from build123d import *

# Parameters (mm, degrees)
SKETCH1_W           = 7.62
SKETCH1_H           = 7.62
BOSS_EXTRUDE1_DEPTH = 10.16
SKETCH2_W           = 7.62
SKETCH2_H           = 7.62
SKETCH2_R           = 1.905
CUT_EXTRUDE1_DEPTH  = 7.62
FILLET1_R           = 2.54
FILLET2_R           = 2.54
FILLET3_R           = 2.54
FILLET4_R           = 2.54


with BuildPart() as part:
    # Sketch1 → Boss-Extrude1 (new body)
    with BuildSketch(Plane(origin=(0, 0, 0), x_dir=(1, 0, 0), z_dir=(0, 1, 0))):
        with Locations((3.81, 3.81)):
            Rectangle(SKETCH1_W, SKETCH1_H)
    extrude(amount=BOSS_EXTRUDE1_DEPTH)

    # Sketch2 → Cut-Extrude1 (cut)
    with BuildSketch(Plane(origin=(0, 10.16, 0), x_dir=(1, 0, 0), z_dir=(0, 1, 0))):
        with Locations((3.81, 3.81)):
            Rectangle(SKETCH2_W, SKETCH2_H)
        with Locations(Location((3.81, 3.81, 0), (0, 0, 270))):
            Circle(SKETCH2_R, mode=Mode.SUBTRACT)
    extrude(amount=-CUT_EXTRUDE1_DEPTH, mode=Mode.SUBTRACT)

    # Fillet1
    fillet1_edges = [part.edges().sort_by_distance(p)[0] for p in [
        (7.62, 1.27, -7.62),
    ]]
    fillet(fillet1_edges, radius=FILLET1_R)

    # Fillet2
    fillet2_edges = [part.edges().sort_by_distance(p)[0] for p in [
        (0, 1.27, -7.62),
    ]]
    fillet(fillet2_edges, radius=FILLET2_R)

    # Fillet3
    fillet3_edges = [part.edges().sort_by_distance(p)[0] for p in [
        (7.62, 1.27, 0),
    ]]
    fillet(fillet3_edges, radius=FILLET3_R)

    # Fillet4
    fillet4_edges = [part.edges().sort_by_distance(p)[0] for p in [
        (0, 1.27, 0),
    ]]
    fillet(fillet4_edges, radius=FILLET4_R)


solid = part.part
Geometry check sheet. Reference: the model listing, model coordinates, mm. A direction names the side the tool comes from. Coordinates: 2 decimals unless noted, no trailing zeros. Order: outer loops, then holes, each group sorted by start corner. A loop starts at its lowest first (then second) coordinate and runs counter-clockwise, first axis right, second up. Notation, with made-up numbers: (-2, -19.75) -> (16, -19.75) arc R28 ccw to (16, 11.25) -> close; hole circle Ø5 at (18.25, 83). An arc over 180 degrees is marked (long way). Use a Markdown table: item, result. Add a question column.
1. Cross-section at D-D (z = -6.75). Enter the section's corners in (x, y), and give its area (3 significant figures).
2. Go/stop test with flat-tipped pins: pin 1 Ø2 at (x, y) = (3, 3.5) entering from +Z; pin 2 Ø1.5 at (x, y) = (1, 8) entering from +Z; pin 3 Ø3 at (y, z) = (3.5, -6.5) entering from -X. Record where each tip stops, or that it passes through.
3. Cross-section at B-B (x = 3.81). Enter the section's corners in (y, z) (3 decimals), and give its area (3 significant figures).
4. Set-up check for faces 1 (the face through (4, 1, 0)), 2 (the face through (5, 2.54, -6)): record each of +Z, -Z, +X, -X, +Y, -Y from which the full face is reachable in a straight line by a thin tool's end or side.
5. Cross-section at A-A (y = 1.25). Enter the section's corners in (x, z).
6. Cross-section at C-C (y = 4.75). Enter the section's corners in (x, z) (3 decimals).
7. Material ranges on L1, parallel to Y at x = 0.5, z = -2.5; L2, parallel to X at y = 1.75, z = -6.5; L3, parallel to X at y = 8, z = -4.75, recorded low to high.
Filled sheet:
| question | item | result |
|---|---|---|
| 1 | outline | (0.63, 0) -> (6.99, 0) -> (6.99, 2.54) -> (0.63, 2.54) -> close |
| 1 | area | 16.2 mm2 |
| 2 | pin 1 | z = 0 |
| 2 | pin 2 | through |
| 2 | pin 3 | x = 0.01 |
| 3 | outline | (0, -7.62) -> (2.54, -7.62) -> (2.54, -5.715) -> (10.16, -5.715) -> (10.16, -1.905) -> (2.54, -1.905) -> (2.54, 0) -> (0, 0) -> close |
| 3 | area | 48.4 mm2 |
| 4 | face 1 | +Z, +X, -X, +Y, -Y |
| 4 | face 2 | +Y |
| 5 | outline | (0, -5.08) arc R2.54 ccw to (2.54, -7.62) -> (5.08, -7.62) arc R2.54 ccw to (7.62, -5.08) -> (7.62, -2.54) arc R2.54 ccw to (5.08, 0) -> (2.54, 0) arc R2.54 ccw to (0, -2.54) -> close |
| 6 | outline | circle Ø3.81 at (3.81, -3.81) |
| 7 | L1 | 0 to 2.54 |
| 7 | L2 | 0.43 to 7.19 |
| 7 | L3 | 2.15 to 5.47 |
